from build123d import *

# Parameters (mm, degrees)
SKETCH1_W           = 60
SKETCH1_H           = 84
BOSS_EXTRUDE1_DEPTH = 33.6
SKETCH2_R           = 1.6
BOSS_EXTRUDE2_DEPTH = 5.8


with BuildPart() as part:
    # Sketch1 → Boss-Extrude1 (new body)
    with BuildSketch(Plane(origin=(0, 0, 0), x_dir=(1, 0, 0), z_dir=(0, 1, 0))):
        Rectangle(SKETCH1_W, SKETCH1_H)
    extrude(amount=BOSS_EXTRUDE1_DEPTH)

    # Sketch2 → Boss-Extrude2 (add)
    with BuildSketch(Plane(origin=(0, 0, 0), x_dir=(1, 0, 0), z_dir=(0, 1, 0))):
        with BuildLine():
            Line((-12.5, 42), (12.5, 42))
            ThreePointArc((12.5, 42), (9.996413035, 42.849853258), (8.527541838, 45.048174357))
            Line((8.527541838, 45.048174357), (6.972458162, 50.851825643))
            ThreePointArc((6.972458162, 50.851825643), (5.503586965, 53.050146742), (3, 53.9))
            Line((3, 53.9), (-3, 53.9))
            ThreePointArc((-3, 53.9), (-5.503586965, 53.050146742), (-6.972458162, 50.851825643))
            Line((-6.972458162, 50.851825643), (-8.527541838, 45.048174357))
            ThreePointArc((-8.527541838, 45.048174357), (-9.996413035, 42.849853258), (-12.5, 42))
        make_face()
        with Locations((0, 48.3)):
            Circle(SKETCH2_R, mode=Mode.SUBTRACT)
        with BuildLine():
            Line((6.972458162, -50.851825643), (8.527541838, -45.048174357))
            ThreePointArc((8.527541838, -45.048174357), (9.996413035, -42.849853258), (12.5, -42))
            Line((12.5, -42), (-12.5, -42))
            ThreePointArc((-12.5, -42), (-9.996413035, -42.849853258), (-8.527541838, -45.048174357))
            Line((-8.527541838, -45.048174357), (-6.972458162, -50.851825643))
            ThreePointArc((-6.972458162, -50.851825643), (-5.503586965, -53.050146742), (-3, -53.9))
            Line((-3, -53.9), (3, -53.9))
            ThreePointArc((3, -53.9), (5.503586965, -53.050146742), (6.972458162, -50.851825643))
        make_face()
        with Locations((0, -48.3)):
            Circle(SKETCH2_R, mode=Mode.SUBTRACT)
    extrude(amount=BOSS_EXTRUDE2_DEPTH)


solid = part.part
Could you check a few things on this model? Use its own coordinates, in mm. A direction names the side the tool comes from. Round coordinates to 2 decimals unless told otherwise and drop trailing zeros. Write each loop counter-clockwise with the first axis right and the second up, starting at its lowest first coordinate (ties: lowest second). Pieces come first, ordered by that corner, then holes. Notation, with made-up numbers: (20, -31) - (62, -31) arc R19 ccw to (62, -10) - close; hole circle Ø8 at (-17, 39). An arc over 180 degrees is marked (long way). Put each result on its own line as item: value. Start each with the question number.
(1) I want a section at A-A, the plane x = 0. Please give me the cut outline in (y, z).
(2) I want a section at D-D, the plane x = 16.5. Please give me the cut outline in (y, z), plus the area to 3 significant figures.
(3) Will these pins go through, and if not, where does the flat tip stop? pin 1 (4 mm diameter, centred on x = 17.5, y = 25, fed in from +Z); pin 2 (12 mm diameter, centred on x = 16, y = 28.5, fed in from -Z); pin 3 (3.5 mm diameter, centred on x = -5.5, z = 49.5, fed in from +Y).
(4) I want a section at B-B, the plane y = 2. Please give me the cut outline in (x, z).
(5) Thinking about a two-plate mould opening in Z: for faces 1 (the flat face through (0, 5.8, -45)), 2 (the cylindrical face through (5.53, 2.86, -53.03)), 3 (the cylindrical face through (0.86, 2.86, 46.95)), which applies, released by +Z, released by -Z, zero draft, split by the parting line, or undercut?
(6) I want a section at C-C, the plane z = -48.3. Please give me the cut outline in (x, y).
(7) For faces 4 (the cylindrical face through (-5.474, 2.859, -53.073)), 5 (the flat face through (-0.2, 5.8, 46.5)), which set-ups out of +Z, -Z, +X, -X, +Y, -Y let a thin tool reach every point of the face, with its end or its side?
(8) I need wall thicknesses on probe 1 along Z at (x, y) = (0, 4); probe 2 along Z at (x, y) = (7, 21.5); probe 3 along X at (y, z) = (1, 48). Which ranges of each line are inside material? Lowest first, please.
Here are the results:
1. outline: (0, -53.9) - (5.8, -53.9) - (5.8, -49.9) - (0, -49.9) - close; (0, -46.7) - (5.8, -46.7) - (5.8, -42) - (33.6, -42) - (33.6, 42) - (5.8, 42) - (5.8, 46.7) - (0, 46.7) - close; (0, 49.9) - (5.8, 49.9) - (5.8, 53.9) - (0, 53.9) - close
2. outline: (0, -42) - (33.6, -42) - (33.6, 42) - (0, 42) - close
2. area: 2,820 mm^2
3. pin 1: stops at z = 42
3. pin 2: stops at z = -42
3. pin 3: stops at y = 5.8
4. outline: (-30, -42) - (-12.5, -42) arc R4.11 cw to (-8.53, -45.05) - (-6.97, -50.85) arc R4.11 ccw to (-3, -53.9) - (3, -53.9) arc R4.11 ccw to (6.97, -50.85) - (8.53, -45.05) arc R4.11 cw to (12.5, -42) - (30, -42) - (30, 42) - (12.5, 42) arc R4.11 cw to (8.53, 45.05) - (6.97, 50.85) arc R4.11 ccw to (3, 53.9) - (-3, 53.9) arc R4.11 ccw to (-6.97, 50.85) - (-8.53, 45.05) arc R4.11 cw to (-12.5, 42) - (-30, 42) - close; hole circle Ø3.2 at (0, -48.3); hole circle Ø3.2 at (0, 48.3)
5. face 1: zero draft
5. face 2: released by -Z
5. face 3: undercut
6. outline: (-7.66, 0) - (-1.6, 0) - (-1.6, 5.8) - (-7.66, 5.8) - close; (1.6, 0) - (7.66, 0) - (7.66, 5.8) - (1.6, 5.8) - close
7. face 4: -Z, -X, +Y, -Y
7. face 5: +Z, +X, -X, +Y
8. probe 1: z = -53.9 to -49.9, -46.7 to 46.7, 49.9 to 53.9
8. probe 2: z = -42 to 42
8. probe 3: x = -7.74 to -1.57, 1.57 to 7.74
